Verification items for the finished model (mm, model axes). A direction names the side the tool comes from. Round coordinates to 2 decimals unless told otherwise and drop trailing zeros. Write each loop counter-clockwise with the first axis right and the second up, starting at its lowest first coordinate (ties: lowest second). Pieces come first, ordered by that corner, then holes. Notation, with made-up numbers: (-13, 35) - (37, 35) arc R19 cw to (37, 61) - close; hole circle Ø4 at (87, 26). An arc over 180 degrees is marked (long way). Answer as a JSON object with one key per item and string values. Group by question number.
1) Mould release check, pull along Y, two halves, no side actions. Record for faces 1 (the cylindrical face through (52.57, 10.75, 8.2)), 2 (the flat face through (-25, 0, 5)), 3 (the flat face through (54, 0, 8)), 4 (the cylindrical face through (23.283, 0.541, 2.465)): +Y half, -Y half, draft (parallel to the pull), parting line (faces both ways), or undercut.
2) Section check B-B (y = 0). Enter the section's corners in (x, z), then the cut area to 3 significant figures.
3) Thickness scan on line 1 (Y direction, x = 25, z = 2.5); line 2 (Y direction, x = -25, z = 1.2); line 3 (Z direction, x = 32, y = 7.5). Record the ranges inside material, lowest first.
4) Go/stop test with flat-tipped pins: pin 1 Ø1.8 at (x, y) = (24.5, -0.5) entering from -Z; pin 2 Ø1 at (y, z) = (9.5, 10.5) entering from -X; pin 3 Ø1 at (x, y) = (-15, 8) entering from -Z. Record where each tip stops, or that it passes through.
5) Section check C-C (x = 25). Enter the section's corners in (y, z), then the cut area to 3 significant figures.
6) Section check A-A (z = 2). Enter the section's corners in (x, y).
7) Set-up check for faces 5 (the cylindrical face through (-53, 0, 2)), 6 (the flat face through (25, 0, 5)): record each of +Z, -Z, +X, -X, +Y, -Y from which the full face is reachable in a straight line by a thin tool's end or side.
8) Section check D-D (x = -1.5). Enter the section's corners in (y, z), then the cut area to 3 significant figures.
```python
from build123d import *

# Parameters (mm, degrees)
SKETCH1_W           = 108
SKETCH1_H           = 24.5
BOSS_EXTRUDE1_DEPTH = 12.5
FILLET1_R           = 5
SKETCH2_R           = 1.8
CUT_EXTRUDE1_DEPTH  = 5
FILLET2_R           = 5
FILLET3_R           = 1


with BuildPart() as part:
    # Sketch1 → Boss-Extrude1 (new body)
    with BuildSketch(Plane.XY):
        Rectangle(SKETCH1_W, SKETCH1_H)
    extrude(amount=BOSS_EXTRUDE1_DEPTH)

    # Fillet1
    fillet1_edges = [part.edges().sort_by_distance(p)[0] for p in [
        (0, -12.25, 0),
        (-54, 0, 0),
        (0, 12.25, 0),
        (54, 0, 0),
    ]]
    fillet(fillet1_edges, radius=FILLET1_R)

    # Sketch2 → Cut-Extrude1 (cut)
    with BuildSketch(Plane(origin=(0, 0, 0), x_dir=(-1, 0, 0), z_dir=(0, 0, -1))):
        with Locations((-25, 0)):
            Circle(SKETCH2_R)
        with Locations((25, 0)):
            Circle(SKETCH2_R)
    extrude(amount=-CUT_EXTRUDE1_DEPTH, mode=Mode.SUBTRACT)

    # Fillet2
    # the kernel refuses this fillet: 5 mm, written as the material it takes off along each edge
    with BuildSketch(Plane(origin=(49, 7.25, 5), x_dir=(0, 1, 0), z_dir=(1, 0, 0))) as fillet2_piece_1_section:
        Polygon((0, 0), (FILLET2_R, 0), (FILLET2_R, -FILLET2_R), (0, -FILLET2_R), align=None)
    fillet2_piece_1 = extrude(amount=FILLET2_R, mode=Mode.PRIVATE)
    fillet2_piece_1 = fillet2_piece_1 - Plane(origin=(49, 7.25, 5), x_dir=(0, -0.7071067811865475, 0.7071067811865475), z_dir=(1, 0, 0)) * Sphere(FILLET2_R, mode=Mode.PRIVATE)
    add(fillet2_piece_1, mode=Mode.SUBTRACT)
    with BuildSketch(Plane(origin=(49, -7.25, 5), x_dir=(1, 0, 0), z_dir=(0, -1, 0))) as fillet2_piece_2_section:
        Polygon((0, 0), (FILLET2_R, 0), (FILLET2_R, -FILLET2_R), (0, -FILLET2_R), align=None)
    fillet2_piece_2 = extrude(amount=FILLET2_R, mode=Mode.PRIVATE)
    fillet2_piece_2 = fillet2_piece_2 - Plane(origin=(49, -7.25, 5), x_dir=(-0.7071067811865475, 0, 0.7071067811865475), z_dir=(0, -1, 0)) * Sphere(FILLET2_R, mode=Mode.PRIVATE)
    add(fillet2_piece_2, mode=Mode.SUBTRACT)
    with BuildSketch(Plane(origin=(-49, 7.25, 5), x_dir=(0, 1, 0), z_dir=(-1, 0, 0))) as fillet2_piece_3_section:
        Polygon((0, 0), (FILLET2_R, 0), (FILLET2_R, FILLET2_R), (0, FILLET2_R), align=None)
    fillet2_piece_3 = extrude(amount=FILLET2_R, mode=Mode.PRIVATE)
    fillet2_piece_3 = fillet2_piece_3 - Plane(origin=(-49, 7.25, 5), x_dir=(0, -0.7071067811865475, 0.7071067811865475), z_dir=(-1, 0, 0)) * Sphere(FILLET2_R, mode=Mode.PRIVATE)
    add(fillet2_piece_3, mode=Mode.SUBTRACT)
    with BuildSketch(Plane(origin=(-49, -7.25, 5), x_dir=(-1, 0, 0), z_dir=(0, -1, 0))) as fillet2_piece_4_section:
        Polygon((0, 0), (FILLET2_R, 0), (FILLET2_R, FILLET2_R), (0, FILLET2_R), align=None)
    fillet2_piece_4 = extrude(amount=FILLET2_R, mode=Mode.PRIVATE)
    fillet2_piece_4 = fillet2_piece_4 - Plane(origin=(-49, -7.25, 5), x_dir=(0.7071067811865475, 0, 0.7071067811865475), z_dir=(0, -1, 0)) * Sphere(FILLET2_R, mode=Mode.PRIVATE)
    add(fillet2_piece_4, mode=Mode.SUBTRACT)
    with BuildSketch(Plane(origin=(54, -12.25, 5), x_dir=(-1, 0, 0), z_dir=(0, 0, 1)), Plane(origin=(54, 12.25, 5), x_dir=(0, -1, 0), z_dir=(0, 0, 1))) as fillet2_piece_5:
        with BuildLine():
            CenterArc((FILLET2_R, -FILLET2_R), FILLET2_R, 90, 90)
            Line((0, -FILLET2_R), (0, 0))
            Line((0, 0), (FILLET2_R, 0))
        make_face()
    extrude(amount=20, mode=Mode.SUBTRACT)
    with BuildSketch(Plane(origin=(-54, -12.25, 5), x_dir=(1, 0, 0), z_dir=(0, 0, 1)), Plane(origin=(-54, 12.25, 5), x_dir=(0, -1, 0), z_dir=(0, 0, 1))) as fillet2_piece_6:
        with BuildLine():
            CenterArc((FILLET2_R, FILLET2_R), FILLET2_R, 180, 90)
            Line((0, FILLET2_R), (0, 0))
            Line((0, 0), (FILLET2_R, 0))
        make_face()
    extrude(amount=20, mode=Mode.SUBTRACT)

    # Fillet3
    fillet3_edges = [part.edges().sort_by_distance(p)[0] for p in [
        (0, -12.25, 12.5),
        (-54, 0, 12.5),
        (54, 0, 12.5),
        (0, 12.25, 12.5),
        (52.535533906, 10.785533906, 12.5),
        (52.535533906, -10.785533906, 12.5),
        (-52.535533906, 10.785533906, 12.5),
        (-52.535533906, -10.785533906, 12.5),
    ]]
    fillet(fillet3_edges, radius=FILLET3_R)


solid = part.part
```
Returned:
{
 "1": {"face 1": "+Y half", "face 2": "undercut", "face 3": "draft", "face 4": "undercut"},
 "2": {"outline": "(-54, 5) arc R5 ccw to (-49, 0) - (-26.8, 0) - (-26.8, 5) - (-23.2, 5) - (-23.2, 0) - (23.2, 0) - (23.2, 5) - (26.8, 5) - (26.8, 0) - (49, 0) arc R5 ccw to (54, 5) - (54, 11.5) arc R1 ccw to (53, 12.5) - (-53, 12.5) arc R1 ccw to (-54, 11.5) - close", "area": "1,300 mm2"},
 "3": {"line 1": "-11.58 to -1.8, 1.8 to 11.58", "line 2": "-10.5 to -1.8, 1.8 to 10.5", "line 3": "0.01 to 12.5"},
 "4": {"pin 1": "z = 5", "pin 2": "x = -53.68", "pin 3": "z = 0.01"},
 "5": {"outline": "(-12.25, 5) arc R5 ccw to (-7.25, 0) - (-1.8, 0) - (-1.8, 5) - (1.8, 5) - (1.8, 0) - (7.25, 0) arc R5 ccw to (12.25, 5) - (12.25, 11.5) arc R1 ccw to (11.25, 12.5) - (-11.25, 12.5) arc R1 ccw to (-12.25, 11.5) - close", "area": "277 mm2"},
 "6": {"outline": "(-53, -7.25) arc R4 ccw to (-49, -11.25) - (49, -11.25) arc R4 ccw to (53, -7.25) - (53, 7.25) arc R4 ccw to (49, 11.25) - (-49, 11.25) arc R4 ccw to (-53, 7.25) - close; hole circle Ø3.6 at (-25, 0); hole circle Ø3.6 at (25, 0)"},
 "7": {"face 5": "-Z, -X, +Y, -Y", "face 6": "-Z"},
 "8": {"outline": "(-12.25, 5) arc R5 ccw to (-7.25, 0) - (7.25, 0) arc R5 ccw to (12.25, 5) - (12.25, 11.5) arc R1 ccw to (11.25, 12.5) - (-11.25, 12.5) arc R1 ccw to (-12.25, 11.5) - close", "area": "295 mm2"}
}
